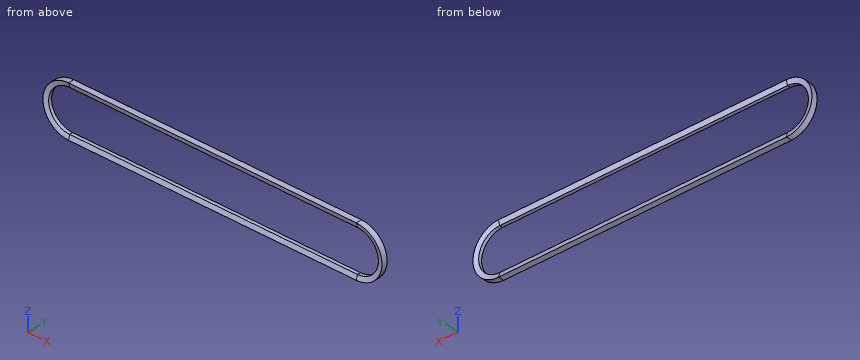
```python
from build123d import *


with BuildPart() as part:
    # Sweep1: sweep along a path in Sketch1
    with BuildLine(Plane(origin=(0, 0, 0), x_dir=(1, 0, 0), z_dir=(0, 1, 0))) as sweep1_path:
        Line((-217.695, 31.75), (217.695, 31.75))
        ThreePointArc((217.695, 31.75), (249.445, 0), (217.695, -31.75))
        Line((217.695, -31.75), (-217.695, -31.75))
        ThreePointArc((-217.695, -31.75), (-249.445, 0), (-217.695, 31.75))
    # Sketch2 → Sweep1 (sweep)
    with BuildSketch(Plane(origin=(0, 0, 0), x_dir=(0, 0, -1), z_dir=(1, 0, 0))):
        Polygon((-38.75, 4.375644347), (-31.75, 2.5), (-31.75, -2.5), (-38.75, -4.375644347), align=None)
    sweep(path=sweep1_path.line)


solid = part.part
```
Build history of the part. All positions in model axes, mm. Give positions to 0.01 mm unless a question says otherwise; leave off trailing zeros. Loops run counter-clockwise (first coordinate to the right, second up) from the corner with the lowest first, then second, coordinate; pieces in that order, holes last. Notation, with made-up numbers: (20.25, 72) - (42.25, 72) arc R20 cw to (42.25, 91) - close; hole circle Ø4 at (54.5, 52.5). An arc over 180 degrees is marked (long way). Use a Markdown table: item, result.
(1) Band-saw the part on C-C (y = -1). Give the cut face in (x, z) (3 decimals).
Taken from the geometry:
| item | result |
|---|---|
| outline | (-217.695, -38.75) - (217.695, -38.75) arc R38.75 ccw to (217.695, 38.75) - (-217.695, 38.75) arc R38.75 ccw to start; hole (-217.695, -31.75) - (217.695, -31.75) arc R31.75 ccw to (217.695, 31.75) - (-217.695, 31.75) arc R31.75 ccw to start |
(2) Wall check: line 1 along Z through (x, y) = (-78, -1); line 2 along X through (y, z) = (1.25, 2.5); line 3 along X through (y, z) = (0.5, 2). Give the ranges that are in metal, low to high.
Taken from the geometry:
| item | result |
|---|---|
| line 1 | -38.75 to -31.75, 31.75 to 38.75 |
| line 2 | -256.36 to -249.35, 249.35 to 256.36 |
| line 3 | -256.39 to -249.38, 249.38 to 256.39 |
(3) Band-saw the part on A-A (x = -43). Give the cut face in (y, z), and give its area (3 significant figures).
Taken from the geometry:
| item | result |
|---|---|
| outline | (-4.38, -38.75) - (4.38, -38.75) - (2.5, -31.75) - (-2.5, -31.75) - close; (-4.38, 38.75) - (-2.5, 31.75) - (2.5, 31.75) - (4.38, 38.75) - close |
| area | 96.3 mm2 |
(4) Band-saw the part on B-B (z = 0). Give the cut face in (x, y) (3 decimals), and give its area (3 significant figures).
Taken from the geometry:
| item | result |
|---|---|
| outline | (-256.445, -4.376) - (-249.445, -2.5) - (-249.445, 2.5) - (-256.445, 4.376) - close; (249.445, -2.5) - (256.445, -4.376) - (256.445, 4.376) - (249.445, 2.5) - close |
| area | 96.3 mm2 |
(5) Drop a flat-ended pin along its axis: pin 1 Ø1 at (y, z) = (3, 30) entering from +X. Give the stop position or say it passes through.
Taken from the geometry:
| item | result |
|---|---|
| pin 1 | x = 242.82 |
